from build123d import *

# Parameters (mm, degrees)
SKETCH_1_W             = 155
SKETCH_1_H             = 9
EXTRUDE_1_DEPTH        = 5
SKETCH_3_W             = 155
SKETCH_3_H             = 5
EXTRUDE_2_DEPTH        = 4.25
EXTRUDE_3_DEPTH        = 5
M3X0_5_1_D             = 2.5
PATTERN_LINEAR_1_COUNT = 49
PATTERN_LINEAR_1_PITCH = 3.141592654
PATTERN_LINEAR_2_COUNT = 8
PATTERN_LINEAR_2_PITCH = 20


with BuildPart() as part:
    # 草圖1 → 填料-伸長1 (new body)
    with BuildSketch(Plane.XY):
        Rectangle(SKETCH_1_W, SKETCH_1_H)
    extrude(amount=EXTRUDE_1_DEPTH)

    # 草圖3 → 填料-伸長2 (add)
    with BuildSketch(Plane(origin=(0, 4.5, 0), x_dir=(1, 0, 0), z_dir=(0, 1, 0))):
        with Locations((0, -2.5)):
            Rectangle(SKETCH_3_W, SKETCH_3_H)
    extrude(amount=EXTRUDE_2_DEPTH)

    # 草圖4 → 填料-伸長3 (add, through all)
    with BuildSketch(Plane.XY):
        Polygon((-76.5, 8.75), (-74.019278088, 8.75), (-74.838211115, 11), (-75.681066973, 11), align=None)
    extrude_3 = extrude(amount=EXTRUDE_3_DEPTH)

    # M3x0.5 螺紋孔1 (through all)
    with Locations(Plane.XY.offset(5)):
        with Locations((-70, 0)):
            m3x0_5_1 = Hole(M3X0_5_1_D / 2)

    # 直線複製排列1: 填料-伸長3 ×49
    with Locations(*[(i * PATTERN_LINEAR_1_PITCH, 0, 0) for i in range(1, PATTERN_LINEAR_1_COUNT)]):
        add(extrude_3)

    # 直線複製排列2: M3x0.5 螺紋孔1 ×8
    with Locations(*[(i * PATTERN_LINEAR_2_PITCH, 0, 0) for i in range(1, PATTERN_LINEAR_2_COUNT)]):
        add(m3x0_5_1, mode=Mode.SUBTRACT)


solid = part.part
For this review, take the finished solid that the model builds, in its own axes (mm). Give positions to 0.01 mm unless a question says otherwise; leave off trailing zeros.
Item 1: For line 1 along Y through (x, z) = (50, 3.15); line 2 along Y through (x, z) = (-30, 3.9); line 3 along Y through (x, z) = (39.5, 4.7), list the stretches that pass through material, from the lowest coordinate up.
Item 2: Insertion check: pin 1 (0.5 mm diameter, centred on x = 52, z = 1.5, fed in from +Y). The pin has a flat end and moves straight along its axis. Give the tip position at first contact, or say it passes through.
Item 3: Take a section at A-A, the plane z = 1.65. Give the number of separate pieces and of enclosed holes in the cut face, and give its area (3 significant figures).
Calculated:
1. line 1: y = -4.5 to -1.25, 1.25 to 11
1. line 2: y = -4.5 to -1.25, 1.25 to 8.75
1. line 3: y = -4.5 to 8.75
2. pin 1: stops at y = 8.75
3. separate pieces: 1
3. enclosed holes: 8
3. area: 2,200 mm2
